Autodesk Fusion 360 part; units mm, degrees
sketch "Sketch1" plane through (0, 0, 0) normal (0, 0, 1) x (1, 0, 0) in component "Component"
  arc A0 (19, 12) -> (0, 12) centre (9.5, 5.5) ccw
  line L0 (19, 10) -> (19, 12)
  line L1 (0, 10) -> (0, 12)
  line L2 (0, 10) -> (19, 10)
  line L3 (8, 10) -> (12, 10)
  line L4 (0.2158, 12.3047) -> (3, 12.3047)
  line L5 (3, 12.3047) -> (3, 15)
  line L6 (16.0158, 12.3047) -> (18.7842, 12.3047)
  line L7 (16.0158, 12.3047) -> (16.0158, 14.9891)
  line L8 (0, 10) -> (19, 10)
  line L9 (19, 10) -> (19, 8)
  line L10 (19, 8) -> (0, 8)
  line L11 (0, 8) -> (0, 10)
  dimension "d36" = 19
extrude "Extrude5" add sketch "Sketch1" along normal blind 12 contours A0 L0 L1 L2 L3 L4 L5 L6 L7 L8 | A0 L6 L7 | A0 L4 L5
extrude "Extrude6" cut sketch "Sketch1" along normal blind 8 contours A0 L6 L7
extrude "Extrude7" add sketch "Sketch1" along normal blind 4 contours A0 L6 L7
extrude "Extrude8" cut sketch "Sketch1" along normal blind 8 contours A0 L4 L5
extrude "Extrude9" add sketch "Sketch1" along normal blind 4 contours A0 L4 L5
extrude "Extrude3" [suppressed] in component "Component"
component "Component" placed x (1, 0, 0) y (0, 1, 0) z (0, 0, 1) at (0, 0, 0)
Source: CAD feature listing. Evaluate the final solid. Frame: model axes, mm. A direction names the side the tool comes from. Give positions to 0.01 mm unless a question says otherwise; leave off trailing zeros. Order: outer loops, then holes, each group sorted by start corner. A loop starts at its lowest first (then second) coordinate and runs counter-clockwise, first axis right, second up. Notation, with made-up numbers: (45, -36.75) -> (51, -36.75) arc R7 ccw to (51, -32.75) -> close; hole circle Ø1 at (47.25, -23.5). An arc over 180 degrees is marked (long way). Use a Markdown table: item, result.
Q1. Section B-B (y = 13.25). Return the cut outline in (x, z).
A:
| item | result |
|---|---|
| outline | (0.99, 0) -> (18.01, 0) -> (18.01, 4) -> (16.02, 4) -> (16.02, 8) -> (18.01, 8) -> (18.01, 12) -> (0.99, 12) -> (0.99, 8) -> (3, 8) -> (3, 4) -> (0.99, 4) -> close |
Q2. Pull-direction query (Z, two-part tool) for faces 4 (the face through (19, 11, 6)), 5 (the face through (16.016, 14, 6)); classes: +Z half, -Z half, draft (parallel to the pull), parting line (faces both ways), or undercut.
A:
| item | result |
|---|---|
| face 4 | draft |
| face 5 | undercut |
Q3. First-contact query: P1, Ø1.4, axis at x = 1, z = 6, coming from the +Y side; P2, Ø1, axis at x = 16.5, y = 13.5, coming from the -Z side; P3, Ø1.3, axis at y = 13, z = 6, coming from the -X side; P4, Ø2, axis at y = 13.5, z = 6, coming from the +X side. Flat tips, straight axial feed; report the tip coordinate or a pass-through.
A:
| item | result |
|---|---|
| P1 | y = 12.3 |
| P2 | z = 0 |
| P3 | x = 3 |
| P4 | x = 16.02 |
Q4. Material intervals for line 1 (X direction, y = 16, z = 5); line 2 (Y direction, x = 13.75, z = 11); line 3 (Y direction, x = 18, z = 10), sorted ascending. Write a range as [from, to].
A:
| item | result |
|---|---|
| line 1 | [4.78, 14.22] |
| line 2 | [10, 16.2] |
| line 3 | [10, 13.26] |
Q5. Access query for faces 1 (the face through (17, 13, 4)), 2 (the face through (2, 13, 4)), 3 (the face through (0, 11, 6)). Directions: +Z, -Z, +X, -X, +Y, -Y. A direction counts if a zero-diameter tool reaches every point of the face in a straight line with its end or side. Return the directions, or none.
A:
| item | result |
|---|---|
| face 1 | +X, +Y |
| face 2 | -X, +Y |
| face 3 | +Z, -Z, -X, +Y, -Y |
Q6. Section C-C (x = 17). Return the cut outline in (y, z), and give its area (3 significant figures).
A:
| item | result |
|---|---|
| outline | (10, 0) -> (14.23, 0) -> (14.23, 4) -> (12.3, 4) -> (12.3, 8) -> (14.23, 8) -> (14.23, 12) -> (10, 12) -> close |
| area | 43.1 mm^2 |
Q7. Section D-D (x = 1.5). Return the cut outline in (y, z).
A:
| item | result |
|---|---|
| outline | (10, 0) -> (13.78, 0) -> (13.78, 4) -> (12.3, 4) -> (12.3, 8) -> (13.78, 8) -> (13.78, 12) -> (10, 12) -> close |
Q8. Section A-A (z = 4.25). Return the cut outline in (x, y), and give its area (3 significant figures).
A:
| item | result |
|---|---|
| outline | (0, 10) -> (19, 10) -> (19, 12) arc R11.51 ccw to (18.78, 12.3) -> (16.02, 12.3) -> (16.02, 14.99) arc R11.51 ccw to (3, 15) -> (3, 12.3) -> (0.22, 12.3) arc R11.51 ccw to (0, 12) -> close |
| area | 96.6 mm^2 |
